Input: part model. Units: mm. Frame: model coordinates. Face numbers are marked on the shaded views. A direction names the side the tool comes from. Coordinates: 2 decimals unless noted, no trailing zeros. Loops run counter-clockwise (first coordinate to the right, second up) from the corner with the lowest first, then second, coordinate; pieces in that order, holes last. Notation, with made-up numbers: (-33, 82.5) - (-19, 82.5) arc R28 cw to (-19, 107.5) - close; hole circle Ø10 at (89.25, -18). An arc over 180 degrees is marked (long way). Use a Markdown table: item, result. Add a question column.
1. Draft query along Y for the marked faces 4, 5, 6 and 7. Return one class per face: released by +Y, released by -Y, zero draft, split by the parting line, or undercut.
2. Section query C-C on z = 25. Return the cut outline in (x, y), then the cut area to 3 significant figures.
3. Contact query for flat-ended pins moving along their axis: P1, Ø10, axis at y = 50.5, z = 24, coming from the -X side; P2, Ø1, axis at y = -86, z = 20.5, coming from the -X side; P3, Ø2, axis at x = -10.5, y = -62.5, coming from the -Z side; P4, Ø3, axis at x = 15.5, y = 15.5, coming from the +Z side. Output: stop coordinate, or through.
4. Section query A-A on y = -2. Return the cut outline in (x, z), then the cut area to 3 significant figures.
5. Ray query, L1, parallel to Z at x = 0, y = -81; L2, parallel to X at y = -12, z = 16; L3, parallel to Z at x = -17, y = -4. Return the intervals inside material, ascending. Write a range as [from, to].
6. Section query B-B on z = 2.5. State how many separate pieces and enclosed holes the cut face has, then the cut area to 3 significant figures.
7. Access query for the marked faces 1, 2 and 3. Directions: +Z, -Z, +X, -X, +Y, -Y. A direction counts if a zero-diameter tool reaches every point of the face in a straight line with its end or side. Return the directions, or none.
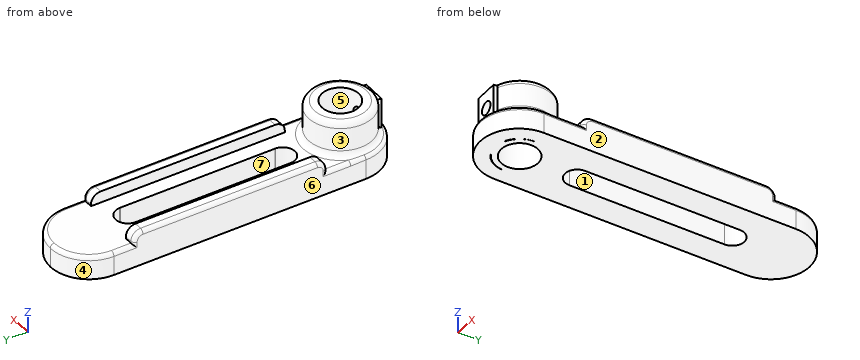
```python
from build123d import *

# Parameters (mm, degrees)
F0_R          = 12.5
F1_DEPTH      = 12
F3_START      = 12
F2_R          = 16.5
F2_R_2        = 12.5
F2_R_3        = 9.5
F3_DEPTH      = 18
F4_DEPTH      = 30
F5_R          = 9.5
F6_DEPTH      = 25
F6_DEPTH_BACK = 100
F7_R          = 3
F9_DEPTH      = 50
F9_DEPTH_BACK = 50
F10_R         = 5
F11_R         = 19.99999
F12_W         = 12
F12_H         = 6
F13_DEPTH     = 28
F15_START     = 70
F14_R         = 3.4
F15_DEPTH     = 30
F16_R         = 2


# Not quite as in the source:
# - a fillet or chamfer is up to 0.001 mm smaller than in the source, because OpenCascade refuses the exact size


with BuildPart() as f1:
    # F0 (on Top) → F1 (new body)
    with BuildSketch(Plane.XY):
        with BuildLine():
            Line((20, -70), (20, 80))
            Line((20, 80), (-20, 80))
            Line((-20, 80), (-20, -70))
            ThreePointArc((-20, -70), (0, -90), (20, -70))
        make_face()
        with Locations((0, -70)):
            Circle(F0_R, mode=Mode.SUBTRACT)
        with BuildLine():
            ThreePointArc((6.2482987692, -40.1458166336), (-0.0729132787, -46.2495746778), (-6.25, -40))
            Line((-6.25, -40), (-6.25, 40))
            ThreePointArc((-6.25, 40), (-0.0729132787, 46.2495746778), (6.2482987692, 40.1458166336))
            ThreePointArc((6.2482987692, 40.1458166336), (6.25, 40), (6.2482987692, 39.8541833664))
            Line((6.2482987692, 39.8541833664), (6.2482987692, -39.8541833664))
            ThreePointArc((6.2482987692, -39.8541833664), (6.25, -40), (6.2482987692, -40.1458166336))
        make_face(mode=Mode.SUBTRACT)
    extrude(amount=F1_DEPTH)

    # F2 (on Top) → F3 (join)
    with BuildSketch(Plane.XY.offset(F3_START)):
        with Locations((0, -69.6852505207)):
            Circle(F2_R)
        with Locations((0, -69.6852505207)):
            Circle(F2_R_2, mode=Mode.SUBTRACT)
        with Locations((0, -69.6852505207)):
            Circle(F2_R_2)
        with Locations((0, -69.6852505207)):
            Circle(F2_R_3, mode=Mode.SUBTRACT)
    extrude(amount=F3_DEPTH)

    # F2 (on Top) → F4 (join)
    with BuildSketch(Plane.XY):
        with Locations((0, -69.6852505207)):
            Circle(F2_R_2)
        with Locations((0, -69.6852505207)):
            Circle(F2_R_3, mode=Mode.SUBTRACT)
        with Locations((0, -69.6852505207)):
            Circle(F2_R_3)
    extrude(amount=F4_DEPTH)

    # F5 (on Top) → F6 (cut, two sides)
    with BuildSketch(Plane.XY) as f6_sk:
        with Locations((0, -69.6852505207)):
            Circle(F5_R)
    extrude(amount=-F6_DEPTH, mode=Mode.SUBTRACT)
    extrude(f6_sk.sketch, amount=F6_DEPTH_BACK, mode=Mode.SUBTRACT)

    # F7
    f7_edges = [f1.edges().sort_by_distance(p)[0] for p in [
        (-16.5, -69.685251, 30),
        (-16.5, -69.685251, 12),
    ]]
    fillet(f7_edges, radius=F7_R)

    # F8 (on Front) → F9 (join, two sides)
    with BuildSketch(Plane.XZ) as f9_sk:
        Polygon((14, 0), (20, 0), (20, 18), (14, 18), (14, 12), align=None)
        Polygon((-14, 0), (-14, 12), (-14, 18), (-20, 18), (-20, 0), align=None)
    extrude(amount=F9_DEPTH)
    extrude(f9_sk.sketch, amount=-F9_DEPTH_BACK)

    # F10
    f10_edges = [f1.edges().sort_by_distance(p)[0] for p in [
        (17, 50, 18),
        (-17, 50, 18),
        (-17, -50, 18),
        (17, -50, 18),
    ]]
    fillet(f10_edges, radius=F10_R)

    # F11 (radius 20 in the source; OpenCascade refuses exactly that, so slightly less here)
    f11_edges = [f1.edges().sort_by_distance(p)[0] for p in [
        (-20, 80, 6),
        (20, 80, 6),
    ]]
    fillet(f11_edges, radius=F11_R)

    # F12 (on Top) → F13 (join)
    with BuildSketch(Plane.XY):
        with Locations((0, -83.9288532734)):
            Rectangle(F12_W, F12_H)
    extrude(amount=F13_DEPTH)

    # F14 (on Front) → F15 (cut)
    with BuildSketch(Plane.XZ.offset(F15_START)):
        with Locations((0, 19)):
            Circle(F14_R)
    extrude(amount=F15_DEPTH, mode=Mode.SUBTRACT)

    # F16
    f16_edges = [f1.edges().sort_by_distance(p)[0] for p in [
        (20, 55.000005, 12),
        (-14.142139, 74.142139, 12),
        (-20, 55.000005, 12),
        (20, -60, 12),
        (-20, -48.535534, 16.535534),
        (-20, 0, 18),
        (20, 0, 18),
        (20, -48.535534, 16.535534),
    ]]
    fillet(f16_edges, radius=F16_R)


solid = f1.part
```
Resolved:
| question | item | result |
|---|---|---|
| 1 | face 4 | released by +Y |
| 1 | face 5 | undercut |
| 1 | face 6 | zero draft |
| 1 | face 7 | undercut |
| 2 | outline | (-6, -86.93) - (6, -86.93) - (6, -85.06) arc R16.5 ccw (long way) to (-6, -85.06) - close; hole circle Ø19 at (0, -69.69) |
| 2 | area | 585 mm² |
| 3 | P1 | through |
| 3 | P2 | x = -6 |
| 3 | P3 | z = 0 |
| 3 | P4 | z = 18 |
| 4 | outline | (-20, 0) - (-6.25, 0) - (-6.25, 12) - (-14, 12) - (-14, 18) - (-18, 18) arc R2 ccw to (-20, 16) - close; (6.25, 0) - (20, 0) - (20, 16) arc R2 ccw to (18, 18) - (14, 18) - (14, 12) - (6.25, 12) - close |
| 4 | area | 400 mm² |
| 5 | L1 | [0, 15.6], [22.4, 30] |
| 5 | L2 | [-20, -14], [14, 20] |
| 5 | L3 | [0, 18] |
| 6 | separate pieces | 1 |
| 6 | enclosed holes | 4 |
| 6 | area | 5,050 mm² |
| 7 | face 1 | +Z, -Z |
| 7 | face 2 | +Z, -Z, +X, +Y, -Y |
| 7 | face 3 | +Z |
